from build123d import *

# Parameters (mm, degrees)
SKETCH1_W           = 100
SKETCH1_H           = 100
SKETCH1_R           = 2.75
BOSS_EXTRUDE1_DEPTH = 14
SKETCH2_R           = 44
SKETCH2_R_2         = 41.4
CUT_EXTRUDE1_DEPTH  = 1.65
SKETCH3_OUTSIDE_W   = 130.422
SKETCH3_OUTSIDE_H   = 130.422
SKETCH3_OUTSIDE_R   = 6.25
CUT_EXTRUDE2_DEPTH  = 73.083285164


with BuildPart() as part:
    # Sketch1 → Boss-Extrude1 (new body)
    with BuildSketch(Plane(origin=(0, 0, 0), x_dir=(1, 0, 0), z_dir=(0, 1, 0))):
        Rectangle(SKETCH1_W, SKETCH1_H)
        with Locations(Location((0, -39, 0), (0, 0, 270))):
            Circle(SKETCH1_R, mode=Mode.SUBTRACT)
        with BuildLine():
            ThreePointArc((7.762235325, 30.064101563), (0, 40), (-7.762235325, 30.064101562))
            ThreePointArc((-7.762235325, 30.064101562), (-13.4720901, 27.975083348), (-18.665386529, 24.813420678))
            ThreePointArc((-18.665386529, 24.813420678), (-31.273259299, 24.939592074), (-28.344735658, 12.675900775))
            ThreePointArc((-28.344735658, 12.675900775), (-30.271511673, 6.909274999), (-31.037591622, 0.877727921))
            ThreePointArc((-31.037591622, 0.877727921), (-38.997116487, -8.900837358), (-27.583071914, -14.257511837))
            ThreePointArc((-27.583071914, -14.257511837), (-24.275867531, -19.359358348), (-20.037857172, -23.718911863))
            ThreePointArc((-20.037857172, -23.718911863), (-17.355349565, -36.038754716), (-6.050792426, -30.454727236))
            ThreePointArc((-6.050792426, -30.454727236), (0, -31.05), (6.050792426, -30.454727236))
            ThreePointArc((6.050792426, -30.454727236), (17.355349565, -36.038754716), (20.037857172, -23.718911863))
            ThreePointArc((20.037857172, -23.718911863), (24.275867531, -19.359358348), (27.583071914, -14.257511837))
            ThreePointArc((27.583071914, -14.257511837), (38.997116487, -8.900837358), (31.037591622, 0.877727921))
            ThreePointArc((31.037591622, 0.877727921), (30.271511673, 6.909274999), (28.344735658, 12.675900775))
            ThreePointArc((28.344735658, 12.675900775), (31.273259299, 24.939592074), (18.665386529, 24.813420678))
            ThreePointArc((18.665386529, 24.813420678), (13.4720901, 27.975083348), (7.762235325, 30.064101563))
        make_face(mode=Mode.SUBTRACT)
    extrude(amount=BOSS_EXTRUDE1_DEPTH)

    # Sketch2 → Cut-Extrude1 (cut)
    with BuildSketch(Plane(origin=(0, 14, 0), x_dir=(1, 0, 0), z_dir=(0, 1, 0))):
        with Locations(Location((0, 0, 0), (0, 0, 270))):
            Circle(SKETCH2_R)
        Circle(SKETCH2_R_2, mode=Mode.SUBTRACT)
    extrude(amount=-CUT_EXTRUDE1_DEPTH, mode=Mode.SUBTRACT)

    # Sketch3 outside → Cut-Extrude2 (cut, through all)
    # profile 1 of 5: a face of its own
    with BuildSketch(Plane(origin=(0, 14, 0), x_dir=(1, 0, 0), z_dir=(0, 1, 0))):
        Rectangle(SKETCH3_OUTSIDE_W, SKETCH3_OUTSIDE_H)
        with BuildLine():
            Line((0, 50), (-37.618424742, 46.708814295))
            ThreePointArc((-37.618424742, 46.708814295), (-43.817935126, 43.817935126), (-46.708814295, 37.618424742))
            Line((-46.708814295, 37.618424742), (-50, 0))
            Line((-50, 0), (-46.708814295, -37.618424742))
            ThreePointArc((-46.708814295, -37.618424742), (-43.817935126, -43.817935126), (-37.618424742, -46.708814295))
            Line((-37.618424742, -46.708814295), (-30.5, -47.331595762))
            ThreePointArc((-30.5, -47.331595762), (0, -44.8), (30.5, -47.331595762))
            Line((30.5, -47.331595762), (37.618424742, -46.708814295))
            ThreePointArc((37.618424742, -46.708814295), (43.817935126, -43.817935126), (46.708814295, -37.618424742))
            Line((46.708814295, -37.618424742), (50, 0))
            Line((50, 0), (46.708814295, 37.618424742))
            ThreePointArc((46.708814295, 37.618424742), (43.817935126, 43.817935126), (37.618424742, 46.708814295))
            Line((37.618424742, 46.708814295), (0, 50))
        make_face(mode=Mode.SUBTRACT)
    # profile 2 of 5: a face of its own
    with BuildSketch(Plane(origin=(0, 14, 0), x_dir=(1, 0, 0), z_dir=(0, 1, 0))):
        with Locations(Location((-38, 38, 0), (0, 0, 270))):
            Circle(SKETCH3_OUTSIDE_R)
    # profile 3 of 5: a face of its own
    with BuildSketch(Plane(origin=(0, 14, 0), x_dir=(1, 0, 0), z_dir=(0, 1, 0))):
        with Locations(Location((38, 38, 0), (0, 0, 90))):
            Circle(SKETCH3_OUTSIDE_R)
    # profile 4 of 5: a face of its own
    with BuildSketch(Plane(origin=(0, 14, 0), x_dir=(1, 0, 0), z_dir=(0, 1, 0))):
        with Locations(Location((38, -38, 0), (0, 0, 270))):
            Circle(SKETCH3_OUTSIDE_R)
    # profile 5 of 5: a face of its own
    with BuildSketch(Plane(origin=(0, 14, 0), x_dir=(1, 0, 0), z_dir=(0, 1, 0))):
        with Locations(Location((-38, -38, 0), (0, 0, 90))):
            Circle(SKETCH3_OUTSIDE_R)
    extrude(amount=-CUT_EXTRUDE2_DEPTH, mode=Mode.SUBTRACT)


solid = part.part
Build history of the part. All positions in model axes, mm. A direction names the side the tool comes from. Coordinates: 2 decimals unless noted, no trailing zeros. Write each loop counter-clockwise with the first axis right and the second up, starting at its lowest first coordinate (ties: lowest second). Pieces come first, ordered by that corner, then holes. Notation, with made-up numbers: (82.5, 25) -> (128.5, 25) arc R16 cw to (128.5, 54) -> close; hole circle Ø10 at (-1, 3.5). An arc over 180 degrees is marked (long way). Use CSV: the item, a comma, the result in double quotes. Start each with the question number.
Q1. Drill centre lines: probe 1 along Z at (x, y) = (-36.5, 10.25); probe 2 along Z at (x, y) = (19.5, 12.75); probe 3 along Z at (x, y) = (-2.5, 13.5). Where is each one in solid material? Low to high.
Q2. Flat gauge pins, fed straight in: pin 1 Ø11 at (x, z) = (38, -38) entering from +Y; pin 2 Ø2 at (x, y) = (23, 11.5) entering from -Z; pin 3 Ø18.5 at (x, z) = (0, -32) entering from -Y; pin 4 Ø4 at (x, y) = (12.5, 7.5) entering from +Z. Where does each tip first touch, or does it go through?
Q3. Cut at B-B, the plane y = 7.25. State how many separate pieces and enclosed holes the cut face has, then the cut area to 3 significant figures.
Q4. Pull direction X, two halves, no side cores. Call faces 1 (the flat face through (-48.33, 7.1, -19.07)), 2 (the cylindrical face through (-0.4, 7.1, 44.8)), 3 (the cylindrical face through (-39.04, 6.9, 8.7)), 4 (the flat face through (34.009, 7.098, 47.025)): released by +X, released by -X, zero draft, split by the parting line, or undercut.
Q5. 3-axis set-ups, long thin cutter, end or side, ignore diameter. For faces 5 (the cylindrical face through (-30.252, 6.902, -6.992)), 6 (the cylindrical face through (-43.887, 7.098, 43.748)): which of +Z, -Z, +X, -X, +Y, -Y reach the whole face in a straight line?
Q6. Cut at A-A, the plane z = 13. List the corners of the cut face in (x, y).
Checked values:
1,probe 1,"z = -46.81 to -44.07, -31.93 to 1.13, 13.11 to 31.93, 44.07 to 46.81"
1,probe 2,"z = -48.29 to -39.44, -36.52 to -25.74, 34.53 to 36.52, 39.44 to 45.83"
1,probe 3,"z = -49.78 to -43.93, -41.32 to -39.6, 30.95 to 37.85, 40.15 to 41.32, 43.93 to 44.82"
2,pin 1,"passes through"
2,pin 2,"stops at z = -48.08"
2,pin 3,"stops at y = 0"
2,pin 4,"stops at z = 45.37"
3,separate pieces,"1"
3,enclosed holes,"6"
3,area,"4,560 mm²"
4,face 1,"released by -X"
4,face 2,"undercut"
4,face 3,"undercut"
4,face 4,"released by +X"
5,face 5,"+Y, -Y"
5,face 6,"+Z, -X, +Y, -Y"
6,outline,"(-48.86, 0) -> (-36.62, 0) -> (-36.62, 14) -> (-39.31, 14) -> (-39.31, 12.35) -> (-42.04, 12.35) -> (-42.04, 14) -> (-48.86, 14) -> close; (36.62, 0) -> (48.86, 0) -> (48.86, 14) -> (42.04, 14) -> (42.04, 12.35) -> (39.31, 12.35) -> (39.31, 14) -> (36.62, 14) -> close"
